from build123d import *

# Parameters (mm, degrees)
SKETCH1_W             = 38.1
SKETCH1_H             = 38.1
SKETCH1_W_2           = 31.75
SKETCH1_H_2           = 31.75
BOSS_EXTRUDE1_DEPTH   = 203.2
SKETCH3_W             = 2.4892
SKETCH3_H             = 38.1
SKETCH3_AT_POINT_2_W  = 2.4892
SKETCH3_AT_POINT_2_H  = 38.1
LPATTERN1_START       = -19.05
LPATTERN1_OUTLINE_R   = 2.4892
LPATTERN1_DEPTH       = 38.1
LPATTERN1_2_OUTLINE_R = 2.4892
LPATTERN1_2_DEPTH     = 38.1


# Read off the part's stored shape, not the designer's step: LPattern1
with BuildPart() as part:
    # Sketch1 → Boss-Extrude1 (new, symmetric)
    with BuildSketch(Plane(origin=(0, 0, 0), x_dir=(0, 0, -1), z_dir=(1, 0, 0))):
        Rectangle(SKETCH1_W, SKETCH1_H)
        Rectangle(SKETCH1_W_2, SKETCH1_H_2, mode=Mode.SUBTRACT)
    extrude(amount=BOSS_EXTRUDE1_DEPTH, both=True)

    # Sketch3 → #9 (0.196) Diameter Hole1 (revolve, cut)
    with BuildSketch(Plane(origin=(190.5, 19.05, 0), x_dir=(0, 0, 1), z_dir=(1, 0, 0))):
        with Locations((1.2446, 19.05)):
            Rectangle(SKETCH3_W, SKETCH3_H)
    revolve(axis=Axis((190.5, 25.4, 0), (0, -1, 0)), mode=Mode.SUBTRACT)

    # Sketch3 at point 2 (carried to point 2, square into its face) → #9 (0.196) Diameter Hole1 at 2 (revolve, cut)
    with BuildSketch(Plane(origin=(190.5, 0, 19.05), x_dir=(0, -1, 0), z_dir=(1, 0, 0))):
        with Locations((1.2446, 19.05)):
            Rectangle(SKETCH3_AT_POINT_2_W, SKETCH3_AT_POINT_2_H)
    revolve(axis=Axis((190.5, 0, 25.4), (0, 0, -1)), mode=Mode.SUBTRACT)

    # LPattern1 outline → LPattern1 (cut)
    with BuildSketch(Plane.XY.offset(LPATTERN1_START)):
        with Locations((165.1, 0)):
            Circle(LPATTERN1_OUTLINE_R)
        with Locations((139.7, 0)):
            Circle(LPATTERN1_OUTLINE_R)
        with Locations((114.3, 0)):
            Circle(LPATTERN1_OUTLINE_R)
        with Locations((88.9, 0)):
            Circle(LPATTERN1_OUTLINE_R)
        with Locations((63.5, 0)):
            Circle(LPATTERN1_OUTLINE_R)
        with Locations((38.1, 0)):
            Circle(LPATTERN1_OUTLINE_R)
        with Locations((12.7, 0)):
            Circle(LPATTERN1_OUTLINE_R)
        with Locations((-12.7, 0)):
            Circle(LPATTERN1_OUTLINE_R)
        with Locations((-38.1, 0)):
            Circle(LPATTERN1_OUTLINE_R)
        with Locations((-63.5, 0)):
            Circle(LPATTERN1_OUTLINE_R)
        with Locations((-88.9, 0)):
            Circle(LPATTERN1_OUTLINE_R)
        with Locations((-114.3, 0)):
            Circle(LPATTERN1_OUTLINE_R)
        with Locations((-139.7, 0)):
            Circle(LPATTERN1_OUTLINE_R)
        with Locations((-165.1, 0)):
            Circle(LPATTERN1_OUTLINE_R)
        with Locations((-190.5, 0)):
            Circle(LPATTERN1_OUTLINE_R)
    extrude(amount=LPATTERN1_DEPTH, mode=Mode.SUBTRACT)

    # LPattern1 2 outline → LPattern1 2 (cut)
    with BuildSketch(Plane(origin=(0, 0, 0), x_dir=(1, 0, 0), z_dir=(0, 1, 0)).offset(LPATTERN1_START)):
        with Locations((165.1, 0)):
            Circle(LPATTERN1_2_OUTLINE_R)
        with Locations((139.7, 0)):
            Circle(LPATTERN1_2_OUTLINE_R)
        with Locations((114.3, 0)):
            Circle(LPATTERN1_2_OUTLINE_R)
        with Locations((88.9, 0)):
            Circle(LPATTERN1_2_OUTLINE_R)
        with Locations((63.5, 0)):
            Circle(LPATTERN1_2_OUTLINE_R)
        with Locations((38.1, 0)):
            Circle(LPATTERN1_2_OUTLINE_R)
        with Locations((12.7, 0)):
            Circle(LPATTERN1_2_OUTLINE_R)
        with Locations((-12.7, 0)):
            Circle(LPATTERN1_2_OUTLINE_R)
        with Locations((-38.1, 0)):
            Circle(LPATTERN1_2_OUTLINE_R)
        with Locations((-63.5, 0)):
            Circle(LPATTERN1_2_OUTLINE_R)
        with Locations((-88.9, 0)):
            Circle(LPATTERN1_2_OUTLINE_R)
        with Locations((-114.3, 0)):
            Circle(LPATTERN1_2_OUTLINE_R)
        with Locations((-139.7, 0)):
            Circle(LPATTERN1_2_OUTLINE_R)
        with Locations((-165.1, 0)):
            Circle(LPATTERN1_2_OUTLINE_R)
        with Locations((-190.5, 0)):
            Circle(LPATTERN1_2_OUTLINE_R)
    extrude(amount=LPATTERN1_2_DEPTH, mode=Mode.SUBTRACT)


solid = part.part
Source: CAD feature listing. Evaluate the final solid. Frame: model axes, mm. A direction names the side the tool comes from. Coordinates: 2 decimals unless noted, no trailing zeros. Order: outer loops, then holes, each group sorted by start corner. A loop starts at its lowest first (then second) coordinate and runs counter-clockwise, first axis right, second up. Notation, with made-up numbers: M 46.5,45 L 93.5,45 A20 ccw 93.5,79 Z; hole C -22,-17.5 d10. An arc over 180 degrees is marked long. Write each question's results on one line, items separated by ' | '. Start each with the question number.
1. Material intervals for L1, parallel to Y at x = 78, z = 15 (3 decimals); L2, parallel to Z at x = 190.5, y = 18.05, sorted ascending.
2. Section B-B, the plane x = 48. Return the cut outline in (y, z) (3 decimals).
3. Pin query (flat end, axial travel): pin 1 (5.5 mm diameter, centred on x = 12.7, z = 0, fed in from +Y). Return the tip coordinate at first contact, or that it passes through.
4. Reachability of faces 1 (the face through (203.2, 0, 17)), 2 (the face through (3, -15.875, 0)) from +Z, -Z, +X, -X, +Y, -Y: full face, straight path, thin tool, end or side. Return the list, or none.
5. Section A-A, the plane y = 6. Return the cut outline in (x, z) (3 decimals), then the cut area to 3 significant figures.
Solution:
1) L1: -19.05 to -15.875, 15.875 to 19.05 | L2: -19.05 to -2.49, 2.49 to 19.05
2) outline: M -19.05,-19.05 L 19.05,-19.05 L 19.05,19.05 L -19.05,19.05 Z; hole M -15.875,-15.875 L 15.875,-15.875 L 15.875,15.875 L -15.875,15.875 Z
3) pin 1: y = 19.05
4) face 1: +Z, -Z, +X, +Y, -Y | face 2: +X, -X
5) outline: M -203.2,-19.05 L 203.2,-19.05 L 203.2,-15.875 L -203.2,-15.875 Z; M -203.2,15.875 L 203.2,15.875 L 203.2,19.05 L -203.2,19.05 Z | area: 2,580 mm²
